Could you check a few things on this model? Use its own coordinates, in mm. Face numbers are marked on the shaded views. A direction names the side the tool comes from. Give positions to 0.01 mm unless a question says otherwise; leave off trailing zeros. Loops run counter-clockwise (first coordinate to the right, second up) from the corner with the lowest first, then second, coordinate; pieces in that order, holes last.
1. Imagine slicing it at A-A (y = 0). List the corners of the cut face in (x, z) for me.
2. For P1, Ø0.9, axis at x = 16, z = 0, coming from the -Y side; P2, Ø4, axis at x = 0, z = 0, coming from the -Y side; P3, Ø5, axis at x = -7.5, y = 1, coming from the +Z side; P4, Ø1.9, axis at x = 0, z = 0, coming from the -Y side, each with a flat end and sliding along its axis, tell me the tip position at first contact or that it passes through.
3. Imagine slicing it at C-C (x = 0). List the corners of the cut face in (y, z) for me.
4. Imagine slicing it at D-D (x = 6.5). List the corners of the cut face in (y, z) for me, plus the area to 3 significant figures.
5. Thinking about a two-plate mould opening in X: for the marked faces 1, 2 and 3, which applies, +X half, -X half, draft (parallel to the pull), parting line (faces both ways), or undercut?
6. For the marked faces 4 and 5, which set-ups out of +Z, -Z, +X, -X, +Y, -Y let a thin tool reach every point of the face, with its end or its side?
7. I need wall thicknesses on line 1 along X through (y, z) = (-3.6, 0); line 2 along X through (y, z) = (13.5, -1.5); line 3 along Y through (x, z) = (5, 2). Which ranges of each line are inside material? Lowest first, please.
8. Imagine slicing it at B-B (z = -15.5). List the corners of the cut face in (x, y) for me, plus the area to 3 significant figures.
```python
from build123d import *

# Parameters (mm, degrees)
SKETCH1_W               = 13.97
SKETCH1_H               = 0.76835
CUT_EXTRUDE1_DEPTH      = 32.597232474
CUT_EXTRUDE1_DEPTH_BACK = 32.597232474
SKETCH2_R               = 1.6
CHAMFER1_SIZE           = 6.35
CUT_EXTRUDE2_DEPTH      = 1.27


with BuildPart() as part:
    # Sketch1 → Revolve1 (revolve)
    with BuildSketch(Plane.XY, mode=Mode.PRIVATE) as revolve1_sk:
        with Locations((6.985, 3.648075)):
            Rectangle(SKETCH1_W, SKETCH1_H)
        Polygon((13.97, 4.03225), (13.97, 3.2639), (16.51, 3.2639), (16.51, 19.05), (13.97, 19.05), align=None)
        with Locations((-6.985, 3.648075)):
            Rectangle(SKETCH1_W, SKETCH1_H)
        Polygon((-16.51, 3.2639), (-13.97, 3.2639), (-13.97, 4.03225), (-13.97, 19.05), (-16.51, 19.05), align=None)
    revolve(revolve1_sk.sketch.rotate(Axis((-15.275524476, 0, 0), (1, 0, 0)), 90), axis=Axis((-15.275524476, 0, 0), (1, 0, 0)))

    # Sketch2 → Cut-Extrude1 (cut, two sides: drawn at the far end of the back side and taken through both)
    with BuildSketch(Plane(origin=(0, 0, 0), x_dir=(1, 0, 0), z_dir=(0, 1, 0)).offset(-CUT_EXTRUDE1_DEPTH_BACK)):
        with Locations(Location((0, 0, 0), (0, 0, 90))):
            Circle(SKETCH2_R)
    extrude(amount=CUT_EXTRUDE1_DEPTH + CUT_EXTRUDE1_DEPTH_BACK, mode=Mode.SUBTRACT)

    # Chamfer1
    chamfer1_edges = [part.edges().sort_by_distance(p)[0] for p in [
        (-13.97, 0, -4.03225),
        (13.97, 0, -4.03225),
    ]]
    chamfer(chamfer1_edges, length=CHAMFER1_SIZE)

    # Sketch3 → Cut-Extrude2 (cut)
    with BuildSketch(Plane(origin=(16.51, 0, 0), x_dir=(0, 0, -1), z_dir=(1, 0, 0))):
        Polygon((-0.720758245, 8.851363919), (0.061967449, 8.851363919), (0.061967449, 4.618030586), (-0.317947081, 4.618030586), (-0.317947081, 8.417175885), (-0.969229132, 8.417175885), align=None)
    extrude(amount=-CUT_EXTRUDE2_DEPTH, mode=Mode.SUBTRACT)


solid = part.part
```
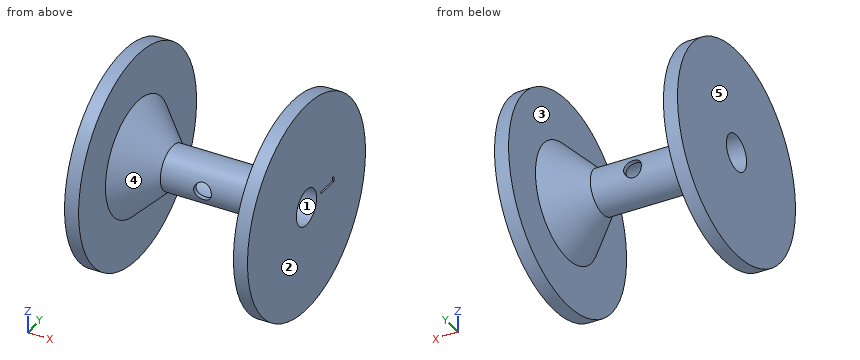
Derived:
1. outline: (-16.51, -19.05) - (-13.97, -19.05) - (-13.97, -10.38) - (-7.62, -4.03) - (7.62, -4.03) - (13.97, -10.38) - (13.97, -19.05) - (16.51, -19.05) - (16.51, -3.26) - (-16.51, -3.26) - close; (-16.51, 3.26) - (16.51, 3.26) - (16.51, 19.05) - (13.97, 19.05) - (13.97, 10.38) - (7.62, 4.03) - (-7.62, 4.03) - (-13.97, 10.38) - (-13.97, 19.05) - (-16.51, 19.05) - close
2. P1: stops at y = -19.05
2. P2: stops at y = -4.03
2. P3: stops at z = 6.36
2. P4: passes through
3. outline: (-3.7, -1.6) arc R4.03 ccw to (3.7, -1.6) - (2.84, -1.6) arc R3.26 cw to (-2.84, -1.6) - close; (-3.7, 1.6) - (-2.84, 1.6) arc R3.26 cw to (2.84, 1.6) - (3.7, 1.6) arc R4.03 ccw to start
4. outline: circle Ø8.06 at (0, 0); hole circle Ø6.53 at (0, 0)
4. area: 17.6 mm2
5. face 1: draft
5. face 2: +X half
5. face 3: undercut
6. face 4: none
6. face 5: +Z, -Z, -X, +Y, -Y
7. line 1: x = -16.51 to -1.6, 1.6 to 16.51
7. line 2: x = -16.51 to -13.97, 13.97 to 16.51
7. line 3: y = -3.5 to -2.58, 2.58 to 3.5
8. outline: (-16.51, -11.07) - (-13.97, -11.07) - (-13.97, 11.07) - (-16.51, 11.07) - close; (13.97, -11.07) - (16.51, -11.07) - (16.51, 11.07) - (13.97, 11.07) - close
8. area: 113 mm2
